Check sheet for the modelled part. Datum: model origin and axes. Units: mm. A direction names the side the tool comes from. Round coordinates to 2 decimals unless told otherwise and drop trailing zeros. Write each loop counter-clockwise with the first axis right and the second up, starting at its lowest first coordinate (ties: lowest second). Pieces come first, ordered by that corner, then holes.
Item 1: Section check D-D, the plane z = -59. Record the cut outline in (x, y).
Item 2: Material ranges on line 1 along Z through (x, y) = (-63, 7.75); line 2 along X through (y, z) = (7.7, -14.5); line 3 along Z through (x, y) = (-56.5, 6.25), recorded low to high.
Item 3: Section check C-C, the plane x = -42.5. Record the cut outline in (y, z).
Item 4: Depth check by flat-ended pin: pin 1 (1 mm diameter, centred on x = -56, y = 8, fed in from +Z); pin 2 (1.5 mm diameter, centred on y = 7, z = -14, fed in from -X); pin 3 (2.5 mm diameter, centred on x = -56.5, z = -74.5, fed in from -Y); pin 4 (5 mm diameter, centred on y = 9.5, z = -39.5, fed in from +X). Enter the tip coordinate at first touch or a pass-through.
Item 5: Set-up check for faces 1 (the flat face through (-32, 11, -77.5)), 2 (the cylindrical face through (0.65, 4.93, -86.07)), 3 (the flat face through (-62.57, 11.48, -80.73)), 4 (the flat face through (-0.4, 11.5, -8.2)): record each of +Z, -Z, +X, -X, +Y, -Y from which the full face is reachable in a straight line by a thin tool's end or side.
Item 6: Section check A-A, the plane z = -89. State how many separate pieces and enclosed holes the cut face has, plus the area to 3 significant figures.
Item 7: Release check for a two-part mould opening along Z. For faces 5 (the flat face through (-55, 5, -13)), 6 (the cylindrical face through (-60, 5, 0)) record: pulls with the +Z half, pulls with the -Z half, needs draft (parallel to the pull), parting line crosses it, or undercut.
Autodesk Inventor part; units mm, degrees
ref_plane "YZ Plane" through (0, 0, 0) normal (1, 0, 0) x (0, 1, 0)
ref_plane "XZ Plane" through (0, 0, 0) normal (0, 1, 0) x (-1, 0, 0)
ref_plane "XY Plane" through (0, 0, 0) normal (0, 0, 1) x (1, 0, 0)
sketch "Sketch1" plane through (0, 0, 0) normal (0, 1, 0) x (-1, 0, 0)
  line L0 (0, 0) -> (63, 0)
  line L1 (63, 0) -> (63, -89)
  line L2 (63, -89) -> (0, -89)
  line L3 (0, -89) -> (0, 0)
  circle A0 centre (0, 0) radius 1.5
  circle A1 centre (63, 0) radius 1.5
  circle A2 centre (0, -89) radius 1.5
  circle A3 centre (63, -89) radius 1.5
  circle A4 centre (0, 0) radius 3
  circle A5 centre (0, -89) radius 3
  circle A6 centre (63, -89) radius 3
  circle A7 centre (63, 0) radius 3
  dimension "d0" = 63
  dimension "d1" = 89
  dimension "d2" = 3
  dimension "d3" = 3
  dimension "d4" = 3
  dimension "d5" = 3
  dimension "d6" = 6
  dimension "d7" = 6
  dimension "d8" = 6
  dimension "d9" = 6
extrude "Extrusion1" add sketch "Sketch1" along normal blind 10 contours A0 L3 A4 L0 | L0 A4 L3 A0 | A7 L1 A1 L0 | L0 A1 L1 A7 | A5 L2 A2 L3 | L3 A2 L2 A5 | A6 L2 A3 L1 | L1 A3 L2 A6
sketch "Sketch2" plane through (0, 10, 0) normal (0, 1, 0) x (1, 0, 0)
  circle A0 centre (0, 0) radius 1.5
  circle A1 centre (-63, 89) radius 1.5
  line L0 (0, 0) -> (-63, 0)
  line L1 (-63, 0) -> (-63, 89)
  line L2 (-63, 89) -> (0, 89)
  line L3 (0, 89) -> (0, 0)
  line L4 (-63, 44.5) -> (-31.5, 44.5)
  line L5 (-6.5, 14.5) -> (-56.5, 14.5)
  line L6 (-56.5, 14.5) -> (-56.5, 74.5)
  line L7 (-56.5, 74.5) -> (-6.5, 74.5)
  line L8 (-6.5, 74.5) -> (-6.5, 14.5)
  line L9 (-6.5, 14.5) -> (-56.5, 74.5) construction
  line L10 (-56.5, 14.5) -> (-6.5, 74.5) construction
  circle A2 centre (-56.5, 14.5) radius 1.5
  circle A3 centre (-6.5, 14.5) radius 1.5
  circle A4 centre (-6.5, 74.5) radius 1.5
  circle A5 centre (-56.5, 74.5) radius 1.5
  circle A6 centre (-56.5, 14.5) radius 3
  circle A7 centre (-56.5, 74.5) radius 3
  circle A8 centre (-6.5, 14.5) radius 3
  circle A9 centre (-6.5, 74.5) radius 3
  dimension "d12" = 50
  dimension "d13" = 60
  dimension "d14" = 3
  dimension "d15" = 3
  dimension "d16" = 3
  dimension "d17" = 3
  dimension "d18" = 6
  dimension "d19" = 6
  dimension "d20" = 6
  dimension "d21" = 6
extrude "Extrusion2" add sketch "Sketch2" against normal blind 5 contours A6 L6 A2 L5 | L5 A2 L6 A6 | A8 L8 A3 L5 | L5 A3 L8 A8 | A9 L7 A4 L8 | L8 A4 L7 A9 | A7 L7 A5 L6 | L6 A5 L7 A7
sketch "Sketch3" plane through (-63, 10, 0) normal (0, 1, 0) x (1, 0, 0)
  circle A0 centre (0, 0) radius 1.5
  circle A1 centre (6.5, 14.5) radius 1.5
  line L0 (0, 0) -> (6.5, 14.5) construction
  line L1 (2.7375, -1.2272) -> (9.2375, 13.2728)
  line L2 (3.7625, 15.7272) -> (-2.7375, 1.2272)
  arc A2 (-2.7375, 1.2272) -> (2.7375, -1.2272) centre (0, 0) ccw
  arc A3 (9.2375, 13.2728) -> (3.7625, 15.7272) centre (6.5, 14.5) ccw
  circle A4 centre (6.5, 74.5) radius 1.5
  line L3 (6.5, 14.5) -> (6.5, 74.5) construction
  line L4 (3.5, 14.5) -> (3.5, 74.5)
  line L5 (9.5, 74.5) -> (9.5, 14.5)
  arc A5 (3.5, 14.5) -> (9.5, 14.5) centre (6.5, 14.5) ccw
  arc A6 (9.5, 74.5) -> (3.5, 74.5) centre (6.5, 74.5) ccw
  circle A7 centre (0, 89) radius 1.5
  line L6 (6.5, 74.5) -> (0, 89) construction
  line L7 (3.7705, 73.2764) -> (-2.7295, 87.7764)
  line L8 (2.7295, 90.2236) -> (9.2295, 75.7236)
  arc A8 (3.7705, 73.2764) -> (9.2295, 75.7236) centre (6.5, 74.5) ccw
  arc A9 (2.7295, 90.2236) -> (-2.7295, 87.7764) centre (0, 89) ccw
  circle A10 centre (63, 89) radius 1.5
  line L9 (0, 89) -> (63, 89) construction
  line L10 (0, 86.0176) -> (63, 86.0176)
  line L11 (63, 91.9824) -> (0, 91.9824)
  arc A11 (0, 91.9824) -> (0, 86.0176) centre (0, 89) ccw
  arc A12 (63, 86.0176) -> (63, 91.9824) centre (63, 89) ccw
  circle A13 centre (56.5, 74.5) radius 1.5
  line L12 (63, 89) -> (56.5, 74.5) construction
  line L13 (60.2705, 90.2236) -> (53.7705, 75.7236)
  line L14 (59.2295, 73.2764) -> (65.7295, 87.7764)
  arc A14 (65.7295, 87.7764) -> (60.2705, 90.2236) centre (63, 89) ccw
  arc A15 (53.7705, 75.7236) -> (59.2295, 73.2764) centre (56.5, 74.5) ccw
  circle A16 centre (56.5, 14.5) radius 1.5
  line L15 (56.5, 74.5) -> (56.5, 14.5) construction
  line L16 (53.5, 74.5) -> (53.5, 14.5)
  line L17 (59.5, 14.5) -> (59.5, 74.5)
  arc A17 (59.5, 74.5) -> (53.5, 74.5) centre (56.5, 74.5) ccw
  arc A18 (53.5, 14.5) -> (59.5, 14.5) centre (56.5, 14.5) ccw
  line L18 (56.5, 14.5) -> (63, 0) construction
  line L19 (53.7705, 13.2764) -> (60.2705, -1.2236)
  line L20 (65.7295, 1.2236) -> (59.2295, 15.7236)
  arc A19 (59.2295, 15.7236) -> (53.7705, 13.2764) centre (56.5, 14.5) ccw
  arc A20 (60.2705, -1.2236) -> (65.7295, 1.2236) centre (63, 0) ccw
  line L21 (63, 0) -> (0, 0) construction
  line L22 (63, 3) -> (0, 3)
  line L23 (0, -3) -> (63, -3)
  arc A21 (63, -3) -> (63, 3) centre (63, 0) ccw
  arc A22 (0, 3) -> (0, -3) centre (0, 0) ccw
  line L24 (6.5, 14.5) -> (56.5, 14.5) construction
  line L25 (6.5, 11.5176) -> (56.5, 11.5176)
  line L26 (56.5, 17.4824) -> (6.5, 17.4824)
  arc A23 (6.5, 17.4824) -> (6.5, 11.5176) centre (6.5, 14.5) ccw
  arc A24 (56.5, 11.5176) -> (56.5, 17.4824) centre (56.5, 14.5) ccw
  line L27 (6.5, 74.5) -> (56.5, 74.5) construction
  line L28 (6.5, 77.5) -> (56.5, 77.5)
  line L29 (56.5, 71.5) -> (6.5, 71.5)
  arc A25 (6.5, 77.5) -> (6.5, 71.5) centre (6.5, 74.5) ccw
  arc A26 (56.5, 71.5) -> (56.5, 77.5) centre (56.5, 74.5) ccw
  circle A27 centre (63, 0) radius 1.5
  circle A28 centre (63, 0) radius 1.5
  circle A29 centre (63, 89) radius 1.5
  circle A30 centre (0, 89) radius 1.5
  point P0 (3.25, 7.25)
  point P1 (6.5, 44.5)
  point P2 (3.25, 81.75)
  point P3 (31.5, 89)
  point P4 (59.75, 81.75)
  point P5 (56.5, 44.5)
  point P6 (59.75, 7.25)
  point P7 (31.5, 0)
  point P8 (31.5, 14.5)
  point P9 (31.5, 74.5)
  point P10 (0.2294, 91.9824)
  point P11 (3.5, 73.8799)
  point P12 (3.5, 15.1417)
  point P13 (65.6357, 1.4329)
  point P14 (59.5, 15.1202)
  point P15 (59.5, 73.8799)
  point P16 (62.7706, 91.9824)
  point P17 (54.5589, 11.5176)
  point P18 (58.3772, 3)
  point P19 (4.6325, 3)
  point P20 (8.4507, 11.5176)
  point P21 (53.5, 17.4824)
  point P22 (9.5, 17.4824)
  point P23 (9.5, 71.5)
  point P24 (53.5, 71.5)
  point P25 (4.6149, 86.0176)
  point P26 (58.3851, 86.0176)
  point P27 (54.5669, 77.5)
  point P28 (8.4331, 77.5)
  point P29 (3.5, 22.3126)
  point P30 (9.5, 14.5)
  point P31 (9.1353, 75.9335)
  point P32 (53.8647, 75.9335)
  point P33 (53.8643, 13.0671)
  point P34 (7.8263, -3)
  point P35 (14.3193, 11.5176)
  point P36 (6.8244, 17.4824)
  point P37 (56.2706, 17.4824)
  point P38 (3.6764, 73.4864)
  point P39 (6.2021, 82.4768)
  point P40 (56.7979, 82.4768)
  point P41 (59.3236, 73.4864)
  dimension "d26" = 6
  dimension "d27" = 6
extrude "Extrusion3" add sketch "Sketch3" along normal blind 3 contours A2 A22 L22 L1 | L1 L22 L19 A20 L20 A21 L23 A2 | L22 A22 L2 L4 A5 L25 L1 | L25 A5 L1 | L1 A3 L5 L26 L16 A18 L19 L25 | L22 A21 L20 A20 L19 | L19 L25 A18 L17 L20 A21 L22 | A5 L25 A23 L26 A3 | A5 L4 L2 A3 L26 A23 L25 | L19 A18 L25 | L4 L7 A25 L29 L5 L26 A3 L2 | A3 L26 L5 | L19 A19 L26 A24 L25 A18 | A18 L16 L26 A19 L19 | L25 A24 L26 A19 L20 L17 A18 | L7 A9 L11 A11 L10 L8 L28 A6 L4 | L4 A25 L7 | L20 A19 L26 L16 L29 A26 L14 L17 | A6 L8 A8 L7 A25 | L7 A8 L8 A6 L5 L29 A25 | L17 A17 L28 L13 L10 A12 L11 A14 L14 | L14 A26 L17 | L5 A6 L8 L28 L13 A17 L16 L29 | L28 L8 A6 | L11 A14 L13 L10 L8 A9 | A9 L8 L10 A11 L11 | A26 L29 L16 A17 L13 A15 L14 | L14 A15 L13 A17 A26 | L11 A12 L10 L13 A14 | A17 L13 L28
properties part number "RP_mounting_cover"
Values found:
1. outline: (-59.5, 10) - (-53.5, 10) - (-53.5, 13) - (-59.5, 13) - close; (-9.5, 10) - (-3.5, 10) - (-3.5, 13) - (-9.5, 13) - close
2. line 1: z = -92 to -90.5, -87.5 to -86, -3 to -1.5, 1.5 to 3
2. line 2: x = -59.5 to -58, -55 to -53.5, -9.5 to -8, -5 to -3.5
2. line 3: z = -77.5 to -76, -73 to -71.5, -17.5 to -16, -13 to -11.5
3. outline: (10, -91.98) - (13, -91.98) - (13, -86.02) - (10, -86.02) - close; (10, -77.5) - (13, -77.5) - (13, -71.5) - (10, -71.5) - close; (10, -17.48) - (13, -17.48) - (13, -11.52) - (10, -11.52) - close; (10, -3) - (13, -3) - (13, 3) - (10, 3) - close
4. pin 1: stops at z = -11.5
4. pin 2: stops at x = -59.5
4. pin 3: passes through
4. pin 4: stops at x = -3.5
5. face 1: +Y, -Y
5. face 2: -Y
5. face 3: -X, +Y, -Y
5. face 4: +X, +Y, -Y
6. separate pieces: 3
6. enclosed holes: 0
6. area: 249 mm2
7. face 5: needs draft
7. face 6: undercut
